```python
from build123d import *

# Parameters (mm, degrees)
PAD_DEPTH    = 22
SKETCH001_R  = 5
PAD001_DEPTH = 17
POCKET_DEPTH = 17


with BuildPart() as part:
    # Sketch → Pad (new body)
    with BuildSketch(Plane.XY):
        with BuildLine():
            ThreePointArc((-7, 0), (0, -7), (7, 0))
            Line((7, 0), (70, 0))
            ThreePointArc((-70, 0), (0, -70), (70, 0))
            Line((-70, 0), (-7, 0))
        make_face()
    extrude(amount=PAD_DEPTH)

    # Sketch001 (on Face6 of Pad) → Pad001 (join)
    with BuildSketch(Plane.XY.offset(22)):
        with Locations((-38.890873, -38.890873)):
            Circle(SKETCH001_R)
        with Locations((38.890873, -38.890873)):
            Circle(SKETCH001_R)
        with Locations((-38.8909, -15)):
            Circle(SKETCH001_R)
        with Locations((38.8909, -15)):
            Circle(SKETCH001_R)
    extrude(amount=-PAD001_DEPTH)

    # Sketch001 (on Face6 of Pad) → Pocket (cut)
    with BuildSketch(Plane.XY.offset(22)):
        with Locations((-38.890873, -38.890873)):
            Circle(SKETCH001_R)
        with Locations((38.890873, -38.890873)):
            Circle(SKETCH001_R)
        with Locations((-38.8909, -15)):
            Circle(SKETCH001_R)
        with Locations((38.8909, -15)):
            Circle(SKETCH001_R)
    extrude(amount=-POCKET_DEPTH, mode=Mode.SUBTRACT)


solid = part.part
```
Design review of the part built by this model. Coordinates are the model's own, in mm. A direction names the side the tool comes from. Coordinates: 2 decimals unless noted, no trailing zeros. Loops run counter-clockwise (first coordinate to the right, second up) from the corner with the lowest first, then second, coordinate; pieces in that order, holes last. Notation, with made-up numbers: M 67,15 L 85,15 A29 cw 85,43 Z; hole C -21,54 d10. An arc over 180 degrees is marked long. One line per question, with ' | ' between items.
(1) Draft analysis for pull direction X (two halves, no side actions). For faces 3 (the face through (38, 0, 11)), 4 (the face through (-34.272, -40.806, 13.619)), 5 (the face through (-1.539, -69.983, 10.846)), state which applies: released by +X, released by -X, zero draft, split by the parting line, or undercut.
Filled in:
face 3: zero draft | face 4: undercut | face 5: split by the parting line
(2) We need section A-A (z = 8.25). Give the boundary of the cut face in (x, y).
Filled in:
outline: M -70,0 A70 ccw 70,0 L 7,0 A7 cw -7,0 Z; hole C -38.89,-38.89 d10; hole C -38.89,-15 d10; hole C 38.89,-38.89 d10; hole C 38.89,-15 d10
(3) We need section D-D (y = -30.5). Give the boundary of the cut face in (x, z).
Filled in:
outline: M -63.01,0 L 63.01,0 L 63.01,22 L -63.01,22 Z
(4) For pin 1 Ø5 at (x, y) = (39.5, -38.5) entering from +Z; pin 2 Ø8 at (y, z) = (-31, 7.5) entering from -X; pin 3 Ø12 at (y, z) = (-36, 7) entering from -X, all flat-tipped, find the tip position at first contact; note any pin that passes through.
Filled in:
pin 1: stops at z = 5 | pin 2: stops at x = -64.58 | pin 3: stops at x = -63.25
(5) Wall thickness on probe 1 along X at (y, z) = (-42, 10); probe 2 along X at (y, z) = (-41, 17.25); probe 3 along Y at (x, z) = (-55.5, 8.5): over which ranges is each line inside the solid? List them lowest first.
Filled in:
probe 1: x = -56 to -42.81, -34.98 to 34.98, 42.81 to 56 | probe 2: x = -56.74 to -43.42, -34.36 to 34.36, 43.42 to 56.74 | probe 3: y = -42.66 to 0
(6) Machinability: for faces 1 (the face through (-39, 0, 11)), 2 (the face through (-34.272, -16.915, 13.619)), which of the approach directions +Z, -Z, +X, -X, +Y, -Y give a long, thin tool a straight path to every point of the face, cutting with its end or side? Answer none if there is none.
Filled in:
face 1: +Z, -Z, +X, -X, +Y | face 2: +Z
(7) We need section B-B (y = -15). Give the boundary of the cut face in (x, z).
Filled in:
outline: M -68.37,0 L 68.37,0 L 68.37,22 L 43.89,22 L 43.89,5 L 33.89,5 L 33.89,22 L -33.89,22 L -33.89,5 L -43.89,5 L -43.89,22 L -68.37,22 Z
(8) We need section C-C (x = 0). Give the boundary of the cut face in (y, z).
Filled in:
outline: M -70,0 L -7,0 L -7,22 L -70,22 Z
